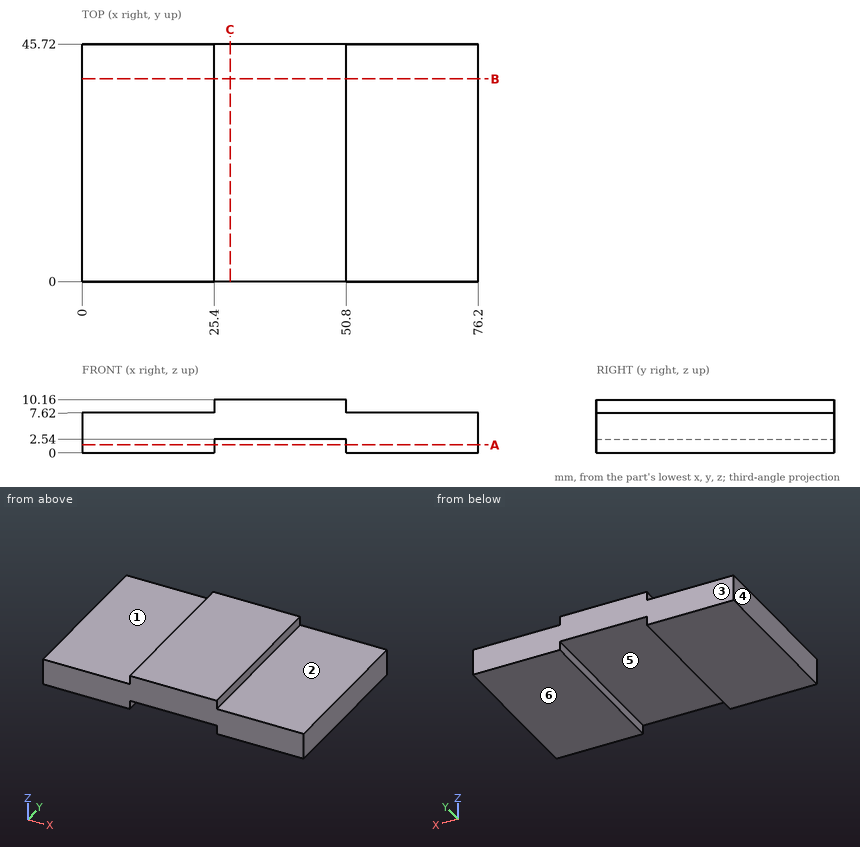
Job drawing, mm, ordinate dimensions from the low corner. One solid piece. A direction names the side the tool comes from. Coordinates: 2 decimals unless noted, no trailing zeros. Write each loop counter-clockwise with the first axis right and the second up, starting at its lowest first coordinate (ties: lowest second). Pieces come first, ordered by that corner, then holes. Notation, with made-up numbers: (-9.5, 79) - (3.5, 79) arc R18 cw to (3.5, 103) - close; hole circle Ø11 at (-14, -34). An arc over 180 degrees is marked (long way). Use a Markdown table: item, result. Add a question column.
Item 1: Mould opens along X. For the marked faces 4, 5 and 6 say: pulls with the +X half, pulls with the -X half, needs draft (parallel to the pull), parting line crosses it, or undercut.
Item 2: Flat gauge pins, fed straight in: pin 1 (12 mm diameter, centred on x = 68, y = 33, fed in from +Z); pin 2 (0.8 mm diameter, centred on y = 25, z = 8.5, fed in from -X); pin 3 (0.8 mm diameter, centred on y = 25, z = 8.5, fed in from +X). Where does each tip first touch, or does it go through?
Item 3: Band-saw the part on C-C, the plane x = 28.5. Give the cut face in (y, z).
Item 4: 3-axis set-ups, long thin cutter, end or side, ignore diameter. For the marked faces 1, 2 and 3: which of +Z, -Z, +X, -X, +Y, -Y reach the whole face in a straight line?
Item 5: Drill centre lines: L1, parallel to X at y = 18.5, z = 1; L2, parallel to Z at x = 55.5, y = 41; L3, parallel to X at y = 11, z = 9. Where is each one in solid material? Low to high. Write a range as from..to.
Item 6: Band-saw the part on B-B, the plane y = 39. Give the cut face in (x, z).
Item 7: Band-saw the part on A-A, the plane z = 1.5. Give the cut face in (x, y).
Numbers:
| question | item | result |
|---|---|---|
| 1 | face 4 | pulls with the -X half |
| 1 | face 5 | undercut |
| 1 | face 6 | needs draft |
| 2 | pin 1 | z = 7.62 |
| 2 | pin 2 | x = 25.4 |
| 2 | pin 3 | x = 50.8 |
| 3 | outline | (0, 2.54) - (45.72, 2.54) - (45.72, 10.16) - (0, 10.16) - close |
| 4 | face 1 | +Z, -X, +Y, -Y |
| 4 | face 2 | +Z, +X, +Y, -Y |
| 4 | face 3 | +Z, -Z, +X, -X, +Y |
| 5 | L1 | 0..25.4, 50.8..76.2 |
| 5 | L2 | 0..7.62 |
| 5 | L3 | 25.4..50.8 |
| 6 | outline | (0, 0) - (25.4, 0) - (25.4, 2.54) - (50.8, 2.54) - (50.8, 0) - (76.2, 0) - (76.2, 7.62) - (50.8, 7.62) - (50.8, 10.16) - (25.4, 10.16) - (25.4, 7.62) - (0, 7.62) - close |
| 7 | outline | (0, 0) - (25.4, 0) - (25.4, 45.72) - (0, 45.72) - close; (50.8, 0) - (76.2, 0) - (76.2, 45.72) - (50.8, 45.72) - close |
